Work out the finished part from the listing and answer in its coordinate system (mm). A direction names the side the tool comes from. Round coordinates to 2 decimals unless told otherwise and drop trailing zeros. Write each loop counter-clockwise with the first axis right and the second up, starting at its lowest first coordinate (ties: lowest second). Pieces come first, ordered by that corner, then holes. Notation, with made-up numbers: M -8,-25 L 24,-25 A19 ccw 24,3 Z; hole C 32.25,34.5 d11. An arc over 180 degrees is marked long. Answer in a Markdown table with one row per item.
Autodesk Inventor part; units mm, degrees
ref_plane "YZ Plane" through (0, 0, 0) normal (1, 0, 0) x (0, 1, 0)
ref_plane "XZ Plane" through (0, 0, 0) normal (0, 1, 0) x (-1, 0, 0)
ref_plane "XY Plane" through (0, 0, 0) normal (0, 0, 1) x (1, 0, 0)
sketch "Sketch1" plane through (0, 0, 0) normal (0, 1, 0) x (-1, 0, 0)
  line L0 (101.6, 101.6) -> (-101.6, 101.6)
  line L1 (-101.6, 101.6) -> (-101.6, -101.6)
  line L2 (-101.6, -101.6) -> (101.6, -101.6)
  line L3 (101.6, -101.6) -> (101.6, 101.6)
  line L4 (101.6, 101.6) -> (-101.6, -101.6) construction
  line L5 (-101.6, 101.6) -> (101.6, -101.6) construction
  point P0 (0, 0)
  dimension "d0" = 203.2
  dimension "d1" = 203.2
extrude "Extrusion1" add sketch "Sketch1" against normal blind 25.4
sketch "Sketch2" plane through (0, 0, 0) normal (0, 1, 0) x (1, 0, 0)
  line L0 (-101.6, -101.6) -> (-101.6, 101.6)
  line L1 (101.6, -101.6) -> (-101.6, -101.6)
  line L2 (-101.6, 101.6) -> (-76.2, 101.6)
  line L3 (-76.2, 101.6) -> (-76.2, -101.6)
  line L4 (-76.2, -101.6) -> (-101.6, -101.6)
  line L5 (-101.6, -101.6) -> (-101.6, 101.6)
  line L6 (101.6, 101.6) -> (101.6, -101.6)
  line L7 (101.6, 101.6) -> (76.2, 101.6)
  line L8 (76.2, 101.6) -> (76.2, -101.6)
  line L9 (76.2, -101.6) -> (101.6, -101.6)
  line L10 (101.6, -101.6) -> (101.6, 101.6)
  point P0 (0, 0)
  dimension "d4" = 25.4
  dimension "d5" = 25.4
extrude "Extrusion2" add sketch "Sketch2" along normal blind 254
sketch "Sketch3" plane through (-101.6, -25.4, -101.6) normal (-1, 0, 0) x (0, 0, 1)
  circle A0 centre (101.6, 254) radius 12.7
  line L0 (0, 279.4) -> (203.2, 279.4)
  point P0 (101.6, 25.4)
  dimension "d8" = 25.4
  dimension "d9" = 25.4
extrude "Extrusion4" cut sketch "Sketch3" against normal through all
properties part number "clutch02-forkBase" material "Wood (Birch)"
1. A tool of negligible diameter and unlimited length cuts with its end or side. For faces 1 (the flat face through (76.2, 125, -1)), 2 (the flat face through (-89, 254, -1)), from which of +Z, -Z, +X, -X, +Y, -Y can it reach the whole face along a straight path? Write none if from no direction.
Calculated:
| item | result |
|---|---|
| face 1 | +Z, -Z, +Y |
| face 2 | +Z, -Z, +X, -X, +Y |
2. The part is cut by section D-D (z = -57.5). Determine the outline of the cut face in (x, y), plus the area to 3 significant figures.
Calculated:
| item | result |
|---|---|
| outline | M -101.6,-25.4 L 101.6,-25.4 L 101.6,254 L 76.2,254 L 76.2,0 L -76.2,0 L -76.2,254 L -101.6,254 Z |
| area | 18,100 mm² |
3. The part is cut by section B-B (z = 0). Determine the outline of the cut face in (x, y).
Calculated:
| item | result |
|---|---|
| outline | M -101.6,-25.4 L 101.6,-25.4 L 101.6,215.9 L 76.2,215.9 L 76.2,0 L -76.2,0 L -76.2,215.9 L -101.6,215.9 Z; M -101.6,241.3 L -76.2,241.3 L -76.2,254 L -101.6,254 Z; M 76.2,241.3 L 101.6,241.3 L 101.6,254 L 76.2,254 Z |
4. The part is cut by section A-A (y = 228.6). Determine the outline of the cut face in (x, z), plus the area to 3 significant figures.
Calculated:
| item | result |
|---|---|
| outline | M -101.6,-101.6 L -76.2,-101.6 L -76.2,-12.7 L -101.6,-12.7 Z; M -101.6,12.7 L -76.2,12.7 L -76.2,101.6 L -101.6,101.6 Z; M 76.2,-101.6 L 101.6,-101.6 L 101.6,-12.7 L 76.2,-12.7 Z; M 76.2,12.7 L 101.6,12.7 L 101.6,101.6 L 76.2,101.6 Z |
| area | 9,030 mm² |
5. Given pin 1 (2 mm diameter, centred on x = -53, z = -5.5, fed in from +Y), flat-ended and moving along its own axis, determine where the tip first touches the part or whether it passes through.
Calculated:
| item | result |
|---|---|
| pin 1 | stops at y = 0 |
6. Determine the mould class of faces 3 (the flat face through (1, 0, 1)), 4 (the flat face through (-83, 74, 101.6)), 5 (the flat face through (-101.6, 116, -1)) for opening direction X: released by +X, released by -X, zero draft, split by the parting line, or undercut.
Calculated:
| item | result |
|---|---|
| face 3 | undercut |
| face 4 | zero draft |
| face 5 | released by -X |
7. Consider line 1 along X through (y, z) = (125, -9); line 2 along Y through (x, z) = (92.5, 0); line 3 along Z through (x, y) = (84, 228). Determine where each line is inside the solid, lowest interval first. Write a range as from..to.
Calculated:
| item | result |
|---|---|
| line 1 | x = -101.6..-76.2, 76.2..101.6 |
| line 2 | y = -25.4..215.9, 241.3..254 |
| line 3 | z = -101.6..-12.69, 12.69..101.6 |
8. The part is cut by section C-C (y = 130). Determine the outline of the cut face in (x, z).
Calculated:
| item | result |
|---|---|
| outline | M -101.6,-101.6 L -76.2,-101.6 L -76.2,101.6 L -101.6,101.6 Z; M 76.2,-101.6 L 101.6,-101.6 L 101.6,101.6 L 76.2,101.6 Z |
